```python
from build123d import *

# Parameters (mm, degrees)
SKETCH2_W                    = 33.6804
SKETCH2_H                    = 19.05
SKETCH2_R                    = 1.189975692
BASE_FLANGE1_DEPTH           = 3.175
EDGE_FLANGE3_STRIP_W         = 19.05
EDGE_FLANGE3_STRIP_H         = 3.175
EDGE_FLANGE3_STRIP_CUT_DEPTH = 19.05
EDGE_FLANGE3_DEPTH           = 19.05
M5_CLEARANCE_HOLE1_D         = 5.5
EDGE_FLANGE5_STRIP_W         = 19.05
EDGE_FLANGE5_STRIP_H         = 3.175
EDGE_FLANGE5_STRIP_CUT_DEPTH = 19.05
EDGE_FLANGE5_DEPTH           = 19.05
EDGE_FLANGE5_START           = 3.175
EDGE_FLANGE5_PROFILE_R       = 1.708184841
EDGE_FLANGE5_FLAT_DEPTH      = 3.175
M8_CLEARANCE_HOLE1_D         = 9
FILLET2_R                    = 3.175


# Sheet-metal steps are written as plain solids
with BuildPart() as part:
    # Sketch2 → Base-Flange1 (new body)
    with BuildSketch(Plane.XY):
        with Locations((7.3152, 0)):
            Rectangle(SKETCH2_W, SKETCH2_H)
        Circle(SKETCH2_R, mode=Mode.SUBTRACT)
    extrude(amount=-BASE_FLANGE1_DEPTH)

    # Edge-Flange3 strip (across the edge) → Edge-Flange3 strip cut (cut)
    with BuildSketch(Plane(origin=(24.1554, 9.525, -3.175), x_dir=(-1, 0, 0), z_dir=(0, -1, 0))):
        with Locations((-3.175, -1.5875)):
            Rectangle(EDGE_FLANGE3_STRIP_W, EDGE_FLANGE3_STRIP_H)
    extrude(amount=EDGE_FLANGE3_STRIP_CUT_DEPTH, mode=Mode.SUBTRACT)

    # Edge-Flange3 section (across the edge) → Edge-Flange3 (add)
    with BuildSketch(Plane(origin=(24.1554, 9.525, -3.175), x_dir=(-1, 0, 0), z_dir=(0, -1, 0))):
        with BuildLine():
            Line((0, 3.175), (0, 54.16804))
            Line((0, 54.16804), (3.175, 54.16804))
            Line((3.175, 54.16804), (3.175, 3.175))
            ThreePointArc((3.175, 3.175), (4.10493597, 0.92993597), (6.35, 0))
            Line((6.35, 0), (6.35, -3.175))
            ThreePointArc((6.35, -3.175), (1.859871939, -1.315128061), (0, 3.175))
        make_face()
    extrude(amount=EDGE_FLANGE3_DEPTH)

    # M5 Clearance Hole1 (through all)
    with Locations(Plane.XY):
        with Locations((0, 0)):
            Hole(M5_CLEARANCE_HOLE1_D / 2)

    # Edge-Flange5 strip (across the edge) → Edge-Flange5 strip cut (cut)
    with BuildSketch(Plane(origin=(24.1554, -9.525, -57.34304), x_dir=(0, 0, 1), z_dir=(0, 1, 0))):
        with Locations((-6.35, -1.5875)):
            Rectangle(EDGE_FLANGE5_STRIP_W, EDGE_FLANGE5_STRIP_H)
    extrude(amount=EDGE_FLANGE5_STRIP_CUT_DEPTH, mode=Mode.SUBTRACT)

    # Edge-Flange5 bend section (across the edge) → Edge-Flange5 (add)
    with BuildSketch(Plane(origin=(24.1554, -9.525, -57.34304), x_dir=(0, 0, 1), z_dir=(0, 1, 0))):
        with BuildLine():
            Line((-3.175, 3.175), (0, 3.175))
            ThreePointArc((0, 3.175), (0.92993597, 0.92993597), (3.175, 0))
            Line((3.175, 0), (3.175, -3.175))
            ThreePointArc((3.175, -3.175), (-1.315128061, -1.315128061), (-3.175, 3.175))
        make_face()
    extrude(amount=EDGE_FLANGE5_DEPTH)

    # Edge-Flange5 profile (on flange) → Edge-Flange5 flat (add)
    with BuildSketch(Plane(origin=(24.1554, 0, -57.34304), x_dir=(0, 1, 0), z_dir=(0, 0, -1)).offset(EDGE_FLANGE5_START)):
        Polygon((-9.525, 3.175), (9.525, 3.175), (9.525, 43.014170651), (-4.326239915, 56.477027), (-19.2786, 56.477027), (-19.2786, 38.189027), (-9.525, 38.189027), align=None)
        with Locations((-10.1346, 47.333027)):
            Circle(EDGE_FLANGE5_PROFILE_R, mode=Mode.SUBTRACT)
    extrude(amount=-EDGE_FLANGE5_FLAT_DEPTH)

    # M8 Clearance Hole1 (through all)
    with Locations(Plane(origin=(0, 0, -60.51804), x_dir=(-1, 0, 0), z_dir=(0, 0, -1))):
        with Locations((-71.488427, -10.1346)):
            Hole(M8_CLEARANCE_HOLE1_D / 2)

    # Fillet2
    fillet2_edges = [part.edges().sort_by_distance(p)[0] for p in [
        (-9.525, 9.525, -1.5875),
        (62.344427, -9.525, -58.93054),
        (67.169570651, 9.525, -58.93054),
        (-9.525, -9.525, -1.5875),
        (80.632427, -4.326239915, -58.93054),
        (80.632427, -19.2786, -58.93054),
        (62.344427, -19.2786, -58.93054),
    ]]
    fillet(fillet2_edges, radius=FILLET2_R)


solid = part.part
```
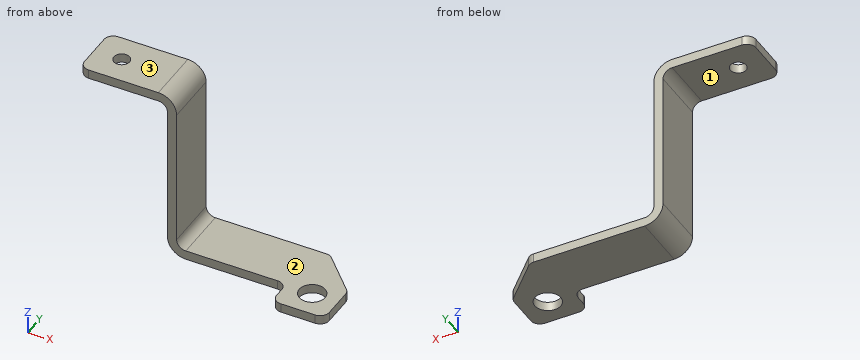
Geometry: final body of the model. Coordinates: model frame, mm. Face numbers are marked on the shaded views. A direction names the side the tool comes from. Coordinates: 2 decimals unless noted, no trailing zeros. Order: outer loops, then holes, each group sorted by start corner. A loop starts at its lowest first (then second) coordinate and runs counter-clockwise, first axis right, second up. Notation, with made-up numbers: (9.25, 88.5) -> (42.25, 88.5) arc R18 ccw to (42.25, 92.5) -> close; hole circle Ø5 at (85.25, -29.75). An arc over 180 degrees is marked (long way). Write each question's results on one line, items separated by ' | '. Start each with the question number.
1) Cut plane C-C, the plane z = -12.5. Output: boundary loops of the cut face in (x, y) (3 decimals), and give its area (3 significant figures).
2) Cut plane A-A, the plane x = 0. Output: boundary loops of the cut face in (y, z) (3 decimals).
3) Set-up query: the marked faces 1, 2 and 3. Return all of +Z, -Z, +X, -X, +Y, -Y with unobstructed straight access to the full face (end or side cutting, diameter ignored); none if empty.
4) Cut plane B-B, the plane y = -8. Output: boundary loops of the cut face in (x, z) (3 decimals), and give its area (3 significant figures).
5) Material intervals for line 1 along Z through (x, y) = (45.5, 2.75); line 2 along X through (y, z) = (-4, -44); line 3 along X through (y, z) = (5.75, -55.5), sorted ascending.
6) First-contact query: pin 1 (15 mm diameter, centred on y = -3, z = -29, fed in from -X); pin 2 (12 mm diameter, centred on x = 19, z = -44.5, fed in from -Y) (3 decimals); pin 3 (11.5 mm diameter, centred on x = 71.49, y = -10.13, fed in from +Z). Flat tips, straight axial feed; report the tip coordinate or a pass-through.
7) Cut plane D-D, the plane x = 73.5. Output: boundary loops of the cut face in (y, z).
Checks:
1) outline: (20.98, -9.525) -> (24.155, -9.525) -> (24.155, 9.525) -> (20.98, 9.525) -> close | area: 60.5 mm^2
2) outline: (-9.525, -3.175) -> (-2.75, -3.175) -> (-2.75, 0) -> (-9.525, 0) -> close; (2.75, -3.175) -> (9.525, -3.175) -> (9.525, 0) -> (2.75, 0) -> close
3) face 1: -Z, -X, +Y, -Y | face 2: +Z, +X, +Y, -Y | face 3: +Z, +X, -X, +Y, -Y
4) outline: (-9.063, -3.175) -> (17.805, -3.175) arc R3.175 cw to (20.98, -6.35) -> (20.98, -54.168) arc R6.35 ccw to (27.33, -60.518) -> (67.527, -60.518) -> (67.527, -57.343) -> (27.33, -57.343) arc R3.175 cw to (24.155, -54.168) -> (24.155, -6.35) arc R6.35 ccw to (17.805, 0) -> (-9.063, 0) -> close; (75.45, -60.518) -> (80.632, -60.518) -> (80.632, -57.343) -> (75.45, -57.343) -> close | area: 429 mm^2
5) line 1: -60.52 to -57.34 | line 2: 20.98 to 24.16 | line 3: 21.12 to 24.45
6) pin 1: x = 20.98 | pin 2: y = -9.525 | pin 3: z = -57.34
7) outline: (-19.28, -60.52) -> (-14.16, -60.52) -> (-14.16, -57.34) -> (-19.28, -57.34) -> close; (-6.11, -60.52) -> (3.01, -60.52) -> (3.01, -57.34) -> (-6.11, -57.34) -> close
